```python
from build123d import *

# Parameters (mm, degrees)
SKETCH1_R           = 75.819
BOSS_EXTRUDE1_DEPTH = 2.0066
SKETCH2_R           = 3.175
CUT_EXTRUDE1_DEPTH  = 108.243032247
CIRPATTERN1_COUNT   = 4


with BuildPart() as part:
    # Sketch1 → Boss-Extrude1 (new body)
    with BuildSketch(Plane.YZ):
        with Locations(Location((0, 0, 0), (0, 0, 270))):
            Circle(SKETCH1_R)
    extrude(amount=BOSS_EXTRUDE1_DEPTH)

    # Sketch2 → Cut-Extrude1 (cut, through all)
    with BuildSketch(Plane.ZY):
        with Locations((63.627, 0)):
            Circle(SKETCH2_R)
    cut_extrude1 = extrude(amount=-CUT_EXTRUDE1_DEPTH, mode=Mode.SUBTRACT)

    # CirPattern1: Cut-Extrude1 ×4 about axis
    cirpattern1_axis = Axis((0, 0, 0), (1, 0, 0))
    for i in range(1, CIRPATTERN1_COUNT):
        add(cut_extrude1.rotate(cirpattern1_axis, i * 360 / CIRPATTERN1_COUNT), mode=Mode.SUBTRACT)


solid = part.part
```
Here's how the part is built. I have some questions about the finished solid (model axes, mm). Round coordinates to 2 decimals unless told otherwise and drop trailing zeros. Order: outer loops, then holes, each group sorted by start corner. A loop starts at its lowest first (then second) coordinate and runs counter-clockwise, first axis right, second up. Notation, with made-up numbers: (54, 82) -> (94, 82) arc R28 cw to (94, 108) -> close; hole circle Ø11 at (16.5, 45). An arc over 180 degrees is marked (long way). Use a Markdown table: item, result. Add a question column.
(1) If we mould it in two halves opening along Y, with no side actions, what happens to faces 1 (the face through (0.99, 1.22, -66.56)), 2 (the face through (0, 1, 1)), 3 (the face through (0.99, -46.13, 60.17)), 4 (the face through (0.99, 66.56, 1.22))? For each: released by +Y, released by -Y, zero draft, split by the parting line, or undercut.
(2) Suppose I cut it at D-D, the plane z = 47.5. Please give me the cut outline in (x, y), and give its area (3 significant figures).
(3) For pin 1 Ø4 at (y, z) = (0, 63.627) entering from +X; pin 2 Ø1 at (x, z) = (0.5, 7.5) entering from +Y, each with a flat end and sliding along its axis, tell me the tip position at first contact or that it passes through.
(4) Suppose I cut it at C-C, the plane x = 0.8. Please give me the cut outline in (y, z) (3 decimals).
(5) I need wall thicknesses on line 1 along Z through (x, y) = (1.65, 18); line 2 along Y through (x, z) = (1.3, 37); line 3 along Z through (x, y) = (1.15, 4.5). Which ranges of each line are inside material? Lowest first, please.
(6) Suppose I cut it at A-A, the plane y = 0. Please give me the cut outline in (x, z), and give its area (3 significant figures).
Verdict:
| question | item | result |
|---|---|---|
| 1 | face 1 | undercut |
| 1 | face 2 | zero draft |
| 1 | face 3 | split by the parting line |
| 1 | face 4 | undercut |
| 2 | outline | (0, -59.1) -> (2.01, -59.1) -> (2.01, 59.1) -> (0, 59.1) -> close |
| 2 | area | 237 mm2 |
| 3 | pin 1 | through |
| 3 | pin 2 | y = 75.5 |
| 4 | outline | circle Ø151.638 at (0, 0); hole circle Ø6.35 at (-63.627, 0); hole circle Ø6.35 at (0, -63.627); hole circle Ø6.35 at (0, 63.627); hole circle Ø6.35 at (63.627, 0) |
| 5 | line 1 | -73.65 to 73.65 |
| 5 | line 2 | -66.18 to 66.18 |
| 5 | line 3 | -75.69 to 75.69 |
| 6 | outline | (0, -75.82) -> (2.01, -75.82) -> (2.01, -66.8) -> (0, -66.8) -> close; (0, -60.45) -> (2.01, -60.45) -> (2.01, 60.45) -> (0, 60.45) -> close; (0, 66.8) -> (2.01, 66.8) -> (2.01, 75.82) -> (0, 75.82) -> close |
| 6 | area | 279 mm2 |
